CAD build for the part. Positions are in the model's coordinates, mm. A direction names the side the tool comes from. Give positions to 0.01 mm unless a question says otherwise; leave off trailing zeros. Write each loop counter-clockwise with the first axis right and the second up, starting at its lowest first coordinate (ties: lowest second). Pieces come first, ordered by that corner, then holes. Notation, with made-up numbers: (32, 63) - (68, 63) arc R7 ccw to (68, 72) - close; hole circle Ø4 at (8, -15.75). An arc over 180 degrees is marked (long way). Answer as a JSON object with one key per item and string values.
from build123d import *

# Parameters (mm, degrees)
EXTRUDE_1_DEPTH     = 10
FILLET_1_R          = 5
SKETCH_2_R          = 2
CUT_EXTRUDE_1_DEPTH = 25.494897428


with BuildPart() as part:
    # 草图1 → 拉伸-薄壁1 (new body)
    with BuildSketch(Plane.XY):
        with BuildLine():
            Line((5, 20), (5, 7))
            ThreePointArc((5, 7), (4.414213562, 5.585786438), (3, 5))
            Line((3, 5), (0, 5))
            ThreePointArc((0, 5), (-5, 0), (0, -5))
            Line((0, -5), (3, -5))
            ThreePointArc((3, -5), (4.414213562, -5.585786438), (5, -7))
            Line((5, -7), (5, -20))
            Line((5, -20), (4, -20))
            Line((4, -20), (4, -7))
            ThreePointArc((4, -7), (3.707106781, -6.292893219), (3, -6))
            Line((3, -6), (0, -6))
            ThreePointArc((0, -6), (-6, 0), (0, 6))
            Line((0, 6), (3, 6))
            ThreePointArc((3, 6), (3.707106781, 6.292893219), (4, 7))
            Line((4, 7), (4, 20))
            Line((4, 20), (5, 20))
        make_face()
    extrude(amount=EXTRUDE_1_DEPTH)

    # 圆角1
    fillet_1_edges = [part.edges().sort_by_distance(p)[0] for p in [
        (4.5, 20, 10),
        (4.5, 20, 0),
        (4.5, -20, 10),
        (4.5, -20, 0),
    ]]
    fillet(fillet_1_edges, radius=FILLET_1_R - 0.0001)  # a hair under: the kernel refuses the full size

    # 草图2 → 切除-拉伸1 (cut, through all)
    with BuildSketch(Plane.ZY.offset(-4)):
        with Locations(Location((5, -15, 0), (0, 0, 270))):
            Circle(SKETCH_2_R)
        with Locations(Location((5, 15, 0), (0, 0, 270))):
            Circle(SKETCH_2_R)
    extrude(amount=-CUT_EXTRUDE_1_DEPTH, mode=Mode.SUBTRACT)


solid = part.part
(1) Probe L1, parallel to Y at x = 2.5, z = 2.75; L2, parallel to Z at x = 4.3, y = 15; L3, parallel to X at y = 17, z = 3.5. List the from-to ranges inside material, lowest first. Write a range as [from, to].
Answer key:
{"L1": "y = [-6, -5], [5, 6]", "L2": "z = [0, 3], [7, 10]", "L3": "x = [4, 5]"}
(2) Pull direction Z, two halves, no side cores. Call faces 6 (the face through (5, 12, 5)), 7 (the face through (4.51, 18.57, 8.5)), 8 (the face through (4.493, 15.26, 6.983)), 9 (the face through (4.49, -18.57, 1.5)): pulls with the +Z half, pulls with the -Z half, needs draft (parallel to the pull), parting line crosses it, or undercut.
Answer key:
{"face 6": "needs draft", "face 7": "pulls with the +Z half", "face 8": "undercut", "face 9": "pulls with the -Z half"}
(3) Saw through at B-B, the plane z = 2.5. Give the cut face in (x, y), and give its area (3 significant figures).
Answer key:
{"outline": "(0, -6) - (3, -6) arc R1 cw to (4, -7) - (4, -19.33) - (5, -19.33) - (5, -7) arc R2 ccw to (3, -5) - (0, -5) arc R5 cw to (0, 5) - (3, 5) arc R2 ccw to (5, 7) - (5, 19.33) - (4, 19.33) - (4, 7) arc R1 cw to (3, 6) - (0, 6) arc R6 ccw to start", "area": "52.7 mm²"}
(4) Saw through at C-C, the plane x = -0.75. Give the cut face in (y, z).
Answer key:
{"outline": "(-5.95, 0) - (-4.94, 0) - (-4.94, 10) - (-5.95, 10) - close; (4.94, 0) - (5.95, 0) - (5.95, 10) - (4.94, 10) - close"}
(5) Saw through at A-A, the plane x = 1. Give the cut face in (y, z), and give its area (3 significant figures).
Answer key:
{"outline": "(-6, 0) - (-5, 0) - (-5, 10) - (-6, 10) - close; (5, 0) - (6, 0) - (6, 10) - (5, 10) - close", "area": "20.0 mm²"}
(6) Saw through at D-D, the plane y = 0. Give the cut face in (x, z).
Answer key:
{"outline": "(-6, 0) - (-5, 0) - (-5, 10) - (-6, 10) - close"}
(7) Flat gauge pins, fed straight in: P1, Ø5, axis at y = 3, z = 9, coming from the +X side; P2, Ø3, axis at y = 15, z = 6.5, coming from the -X side; P3, Ø3.5, axis at x = 2, z = 5, coming from the -Y side. Where does each tip first touch, or does it go through?
Answer key:
{"P1": "stops at x = 4.32", "P2": "stops at x = 4", "P3": "stops at y = -6.34"}
(8) 3-axis set-ups, long thin cutter, end or side, ignore diameter. For faces 1 (the face through (2, 5, 5)), 2 (the face through (4.51, 18.57, 1.5)), 3 (the face through (4, -12, 5)), 4 (the face through (5, -12, 5)), 5 (the face through (4, 12, 5)): which of +Z, -Z, +X, -X, +Y, -Y reach the whole face in a straight line?
Answer key:
{"face 1": "+Z, -Z, +X", "face 2": "-Z, +X, -X, +Y", "face 3": "+Z, -Z, -X, -Y", "face 4": "+Z, -Z, +X, +Y, -Y", "face 5": "+Z, -Z, -X, +Y"}
